from build123d import *

# Parameters (mm, degrees)
SKETCH1_W           = 152.4
SKETCH1_H           = 152.4
BOSS_EXTRUDE1_DEPTH = 12.7
BOSS_EXTRUDE2_DEPTH = 12.7
SKETCH2_R           = 7.62
CUT_EXTRUDE1_DEPTH  = 12.7
FILLET1_R           = 2.54
FILLET2_R           = 2.54


with BuildPart() as part:
    # Sketch1 → Boss-Extrude1 (new body)
    with BuildSketch(Plane.XY):
        Rectangle(SKETCH1_W, SKETCH1_H)
    extrude(amount=BOSS_EXTRUDE1_DEPTH)

    # Sketch3 → Boss-Extrude2 (add)
    with BuildSketch(Plane.ZY.offset(76.2)):
        with BuildLine():
            Line((0, -69.85), (0, -44.45))
            ThreePointArc((0, -44.45), (-12.7, -57.15), (0, -69.85))
        make_face()
    boss_extrude2 = extrude(amount=-BOSS_EXTRUDE2_DEPTH)

    # Sketch2 → Cut-Extrude1 (cut)
    with BuildSketch(Plane.ZY.offset(76.2)):
        with Locations((0, -57.15)):
            Circle(SKETCH2_R)
    cut_extrude1 = extrude(amount=-CUT_EXTRUDE1_DEPTH, mode=Mode.SUBTRACT)

    # Mirror1: Boss-Extrude2, Cut-Extrude1 across plane
    add(boss_extrude2.mirror(Plane(origin=(0, 0, 0), x_dir=(0, 0, 1), z_dir=(1, 0, 0))))
    add(cut_extrude1.mirror(Plane(origin=(0, 0, 0), x_dir=(0, 0, 1), z_dir=(1, 0, 0))), mode=Mode.SUBTRACT)

    # Fillet1
    fillet1_edges = [part.edges().sort_by_distance(p)[0] for p in [
        (0, -76.2, 12.7),
    ]]
    fillet(fillet1_edges, radius=FILLET1_R)

    # Fillet2
    fillet2_edges = [part.edges().sort_by_distance(p)[0] for p in [
        (-76.2, 15.875, 0),
        (-76.2, -57.15, -12.7),
        (-63.5, -57.15, -12.7),
        (76.2, 15.875, 0),
        (63.5, -57.15, -12.7),
        (76.2, -57.15, -12.7),
        (-76.2, 1.27, 12.7),
        (76.2, 1.27, 12.7),
        (76.2, -76.2, 5.08),
        (76.2, -75.456051224, 11.956051224),
        (0, -76.2, 0),
        (-76.2, -76.2, 5.08),
        (-76.2, -75.456051224, 11.956051224),
        (76.2, -73.025, 0),
        (0, 76.2, 0),
        (-76.2, -73.025, 0),
        (0, 76.2, 12.7),
        (76.2, 76.2, 6.35),
        (-76.2, 76.2, 6.35),
    ]]
    fillet(fillet2_edges, radius=FILLET2_R)


solid = part.part
Input: part model. Units: mm. Frame: model coordinates. A direction names the side the tool comes from. Coordinates: 2 decimals unless noted, no trailing zeros. Order: outer loops, then holes, each group sorted by start corner. A loop starts at its lowest first (then second) coordinate and runs counter-clockwise, first axis right, second up. Notation, with made-up numbers: M 2.25,18 L 47.25,18 A20 ccw 47.25,48 Z; hole C -20,33.25 d3. An arc over 180 degrees is marked long. Answer in a Markdown table with one row per item.
(1) Access query for faces 1 (the flat face through (-63.5, -57, 3)), 2 (the flat face through (-63.5, -57, -9)), 3 (the flat face through (63.5, -57, 3)), 4 (the flat face through (-1, -76.2, 6)). Directions: +Z, -Z, +X, -X, +Y, -Y. A direction counts if a zero-diameter tool reaches every point of the face in a straight line with its end or side. Return the directions, or none.
Numbers:
| item | result |
|---|---|
| face 1 | -X |
| face 2 | -Z, +Y, -Y |
| face 3 | +X |
| face 4 | +Z, -Z, +X, -X, -Y |
(2) Draft query along Z for faces 5 (the cylindrical face through (69.939, -49.595, -0.992)), 6 (the flat face through (-1, 1, 12.7)), 7 (the flat face through (-1, 76.2, 6)). Return one class per face: pulls with the +Z half, pulls with the -Z half, needs draft (parallel to the pull), parting line crosses it, or undercut.
Numbers:
| item | result |
|---|---|
| face 5 | undercut |
| face 6 | pulls with the +Z half |
| face 7 | needs draft |
(3) Section query A-A, the plane y = -57.15. Output: boundary loops of the cut face in (x, z).
Numbers:
| item | result |
|---|---|
| outline | M -76.2,-10.16 A2.54 ccw -73.66,-12.7 L -66.04,-12.7 A2.54 ccw -63.5,-10.16 L -63.5,-7.62 L -76.2,-7.62 Z; M -76.2,7.62 L -63.5,7.62 L -63.5,0 L 63.5,0 L 63.5,7.62 L 76.2,7.62 L 76.2,10.16 A2.54 ccw 73.66,12.7 L -73.66,12.7 A2.54 ccw -76.2,10.16 Z; M 63.5,-10.16 A2.54 ccw 66.04,-12.7 L 73.66,-12.7 A2.54 ccw 76.2,-10.16 L 76.2,-7.62 L 63.5,-7.62 Z |
(4) Section query B-B, the plane x = -38.5. Output: boundary loops of the cut face in (y, z), plus the area to 3 significant figures.
Numbers:
| item | result |
|---|---|
| outline | M -76.2,2.54 A2.54 ccw -73.66,0 L 73.66,0 A2.54 ccw 76.2,2.54 L 76.2,10.16 A2.54 ccw 73.66,12.7 L -73.66,12.7 A2.54 ccw -76.2,10.16 Z |
| area | 1,930 mm^2 |
(5) Contact query for flat-ended pins moving along their axis: pin 1 Ø8 at (x, y) = (-27.5, -46.5) entering from -Z; pin 2 Ø12 at (y, z) = (-57.15, 0) entering from +X; pin 3 Ø8 at (y, z) = (-57.5, -5) entering from -X; pin 4 Ø8.5 at (y, z) = (-56, 2) entering from -X. Output: stop coordinate, or through.
Numbers:
| item | result |
|---|---|
| pin 1 | stops at z = 0 |
| pin 2 | stops at x = 63.5 |
| pin 3 | stops at x = -76.2 |
| pin 4 | stops at x = -63.5 |
(6) Section query D-D, the plane z = -4.25. Give the number of separate pieces and of enclosed holes in the cut face, plus the area to 3 significant figures.
Numbers:
| item | result |
|---|---|
| separate pieces | 4 |
| enclosed holes | 0 |
| area | 275 mm^2 |
(7) Material intervals for line 1 (Z direction, x = 72, y = -57); line 2 (Z direction, x = 43.5, y = 14); line 3 (Y direction, x = -41, z = 10.75), sorted ascending. Write a range as [from, to].
Numbers:
| item | result |
|---|---|
| line 1 | z = [-12.7, -7.62], [7.62, 12.7] |
| line 2 | z = [0, 12.7] |
| line 3 | y = [-76.13, 76.13] |
